Design review of the part built by this model. Coordinates are the model's own, in mm. A direction names the side the tool comes from. Coordinates: 2 decimals unless noted, no trailing zeros. Loops run counter-clockwise (first coordinate to the right, second up) from the corner with the lowest first, then second, coordinate; pieces in that order, holes last. Notation, with made-up numbers: (76.5, 60) -> (110.5, 60) arc R6 cw to (110.5, 68) -> close; hole circle Ø10 at (73.25, -11.75). An arc over 180 degrees is marked (long way). One line per item, written item: value. Start each with the question number.
1. Insertion check: pin 1 (5 mm diameter, centred on x = 44.25, y = -2.5, fed in from -Z); pin 2 (1.5 mm diameter, centred on x = -45, y = -66.5, fed in from +Z). Each pin has a flat end and moves straight along its axis. Give the tip position at first contact, or say it passes through.
2. Machinability: for faces 5 (the flat face through (41.75, -3, -7)), 6 (the cylindrical face through (-44.6, -4.06, -8.45)), which of the approach directions +Z, -Z, +X, -X, +Y, -Y give a long, thin tool a straight path to every point of the face, cutting with its end or side? Answer none if there is none.
3. Add section D-D on z = -7.75. Write out the cut boundary in (x, y), plus the area to 3 significant figures.
4. Add section B-B on y = -76. Write out the cut boundary in (x, z), plus the area to 3 significant figures.
5. Add section A-A on x = -29.5. Write out the cut boundary in (y, z).
6. For probe 1 along X at (y, z) = (-67.5, -9.75); probe 2 along X at (y, z) = (-24.5, -8.75); probe 3 along Y at (x, z) = (44.25, -6.75), list the stretches that pass through material, from the lowest coordinate up.
7. Draft analysis for pull direction X (two halves, no side actions). For faces 1 (the flat face through (48.75, -44, -6)), 2 (the flat face through (44, -65, -7)), 3 (the flat face through (-1, -63, -12)), 4 (the flat face through (-48.75, -44, -6)), state which applies: pulls with the +X half, pulls with the -X half, needs draft (parallel to the pull), parting line crosses it, or undercut.
8. Add section C-C on x = 12. Write out the cut boundary in (y, z).
```python
from build123d import *

# Parameters (mm, degrees)
SKETCH001_W     = 97.5
SKETCH001_H     = 91
PAD_DEPTH       = 12
SKETCH_W        = 93.5
SKETCH_H        = 87
POCKET_DEPTH    = 10
SKETCH002_W     = 5
SKETCH002_H     = 5
SKETCH002_R     = 1.6
PAD001_DEPTH    = 10
POCKET001_DEPTH = 5
SKETCH003_W     = 78.5
SKETCH003_H     = 51.5
POCKET002_DEPTH = 12.001
SKETCH004_W     = 45
SKETCH004_H     = 12.5
POCKET003_DEPTH = 12.001
SKETCH005_R     = 1.6
POCKET004_DEPTH = 12.001


with BuildPart() as part:
    # Sketch001 → Pad (new body)
    with BuildSketch(Plane.XY):
        with Locations((0, -43.5)):
            Rectangle(SKETCH001_W, SKETCH001_H)
    extrude(amount=-PAD_DEPTH)

    # Sketch → Pocket (cut)
    with BuildSketch(Plane.XY):
        with Locations((0, -43.5)):
            Rectangle(SKETCH_W, SKETCH_H)
    extrude(amount=-POCKET_DEPTH, mode=Mode.SUBTRACT)

    # Sketch002 → Pad001 (join)
    with BuildSketch(Plane.XY):
        with Locations((-44.25, -2.5)):
            Rectangle(SKETCH002_W, SKETCH002_H)
        with Locations((-44.25, -2.5)):
            Circle(SKETCH002_R, mode=Mode.SUBTRACT)
        with Locations((-44.25, -67.5)):
            Rectangle(SKETCH002_W, SKETCH002_H)
        with Locations((-44.25, -67.5)):
            Circle(SKETCH002_R, mode=Mode.SUBTRACT)
        with Locations((44.25, -67.5)):
            Rectangle(SKETCH002_W, SKETCH002_H)
        with Locations((44.25, -67.5)):
            Circle(SKETCH002_R, mode=Mode.SUBTRACT)
        with Locations((44.25, -2.5)):
            Rectangle(SKETCH002_W, SKETCH002_H)
        with Locations((44.25, -2.5)):
            Circle(SKETCH002_R, mode=Mode.SUBTRACT)
    extrude(amount=-PAD001_DEPTH)

    # Sketch → Pocket001 (cut)
    with BuildSketch(Plane.XY):
        with Locations((0, -43.5)):
            Rectangle(SKETCH_W, SKETCH_H)
    extrude(amount=-POCKET001_DEPTH, mode=Mode.SUBTRACT)

    # Sketch003 → Pocket002 (cut, through all)
    with BuildSketch(Plane.XY):
        with Locations((0, -35.25)):
            Rectangle(SKETCH003_W, SKETCH003_H)
    extrude(amount=-POCKET002_DEPTH, mode=Mode.SUBTRACT)

    # Sketch004 → Pocket003 (cut, through all)
    with BuildSketch(Plane.XY):
        with Locations((-21.25, -78.75)):
            Rectangle(SKETCH004_W, SKETCH004_H)
    extrude(amount=-POCKET003_DEPTH, mode=Mode.SUBTRACT)

    # Sketch005 → Pocket004 (cut, through all)
    with BuildSketch(Plane.XY):
        with Locations((-44.25, -2.5)):
            Circle(SKETCH005_R)
        with Locations((44.25, -2.5)):
            Circle(SKETCH005_R)
        with Locations((44.25, -67.5)):
            Circle(SKETCH005_R)
        with Locations((-44.25, -67.5)):
            Circle(SKETCH005_R)
    extrude(amount=-POCKET004_DEPTH, mode=Mode.SUBTRACT)


solid = part.part
```
Worked answers:
1. pin 1: stops at z = -12
1. pin 2: stops at z = -5
2. face 5: +Z
2. face 6: +Z, -Z
3. outline: (-48.75, -89) -> (48.75, -89) -> (48.75, 2) -> (-48.75, 2) -> close; hole (-46.75, -87) -> (46.75, -87) -> (46.75, -70) -> (41.75, -70) -> (41.75, -65) -> (46.75, -65) -> (46.75, -5) -> (41.75, -5) -> (41.75, 0) -> (-41.75, 0) -> (-41.75, -5) -> (-46.75, -5) -> (-46.75, -65) -> (-41.75, -65) -> (-41.75, -70) -> (-46.75, -70) -> close; hole circle Ø3.2 at (-44.25, -67.5); hole circle Ø3.2 at (-44.25, -2.5); hole circle Ø3.2 at (44.25, -67.5); hole circle Ø3.2 at (44.25, -2.5)
3. area: 806 mm²
4. outline: (-48.75, -12) -> (-43.75, -12) -> (-43.75, -10) -> (-46.75, -10) -> (-46.75, 0) -> (-48.75, 0) -> close; (1.25, -12) -> (48.75, -12) -> (48.75, 0) -> (46.75, 0) -> (46.75, -10) -> (1.25, -10) -> close
4. area: 145 mm²
5. outline: (-89, -12) -> (-85, -12) -> (-85, -10) -> (-87, -10) -> (-87, 0) -> (-89, 0) -> close; (-72.5, -12) -> (-61, -12) -> (-61, -10) -> (-72.5, -10) -> close; (-9.5, -12) -> (2, -12) -> (2, 0) -> (0, 0) -> (0, -10) -> (-9.5, -10) -> close
6. probe 1: x = -48.75 to -45.85, -42.65 to -41.75, 41.75 to 42.65, 45.85 to 48.75
6. probe 2: x = -48.75 to -46.75, 46.75 to 48.75
6. probe 3: y = -89 to -87, -70 to -69.1, -65.9 to -65, -5 to -4.1, -0.9 to 2
7. face 1: pulls with the +X half
7. face 2: undercut
7. face 3: needs draft
7. face 4: pulls with the -X half
8. outline: (-89, -12) -> (-61, -12) -> (-61, -10) -> (-87, -10) -> (-87, 0) -> (-89, 0) -> close; (-9.5, -12) -> (2, -12) -> (2, 0) -> (0, 0) -> (0, -10) -> (-9.5, -10) -> close
